Geometry check sheet. Reference: the model listing, model coordinates, mm. Face numbers are marked on the shaded views. A direction names the side the tool comes from. Give positions to 0.01 mm unless a question says otherwise; leave off trailing zeros. Order: outer loops, then holes, each group sorted by start corner. A loop starts at its lowest first (then second) coordinate and runs counter-clockwise, first axis right, second up.
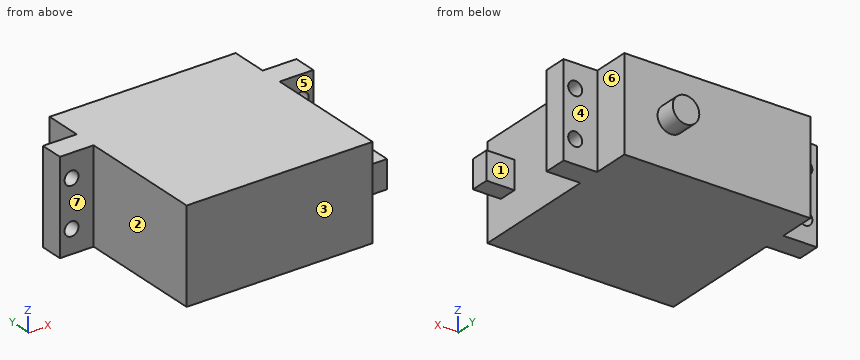
```python
from build123d import *

# Parameters (mm, degrees)
SKETCH1_W           = 40
SKETCH1_H           = 8
SKETCH1_W_2         = 7.25
SKETCH1_H_2         = 5
SKETCH1_H_3         = 27.5
BOSS_EXTRUDE1_DEPTH = 20
SKETCH2_R           = 2.85
BOSS_EXTRUDE2_DEPTH = 4.5
SKETCH3_R           = 1.5
CUT_EXTRUDE1_DEPTH  = 47.891497097
SKETCH4_W           = 6
SKETCH4_H           = 4
BOSS_EXTRUDE3_DEPTH = 6


with BuildPart() as part:
    # Sketch1 → Boss-Extrude1 (new body)
    with BuildSketch(Plane.XY):
        with Locations((0, -4)):
            Rectangle(SKETCH1_W, SKETCH1_H)
        with Locations((-23.625, -10.5)):
            Rectangle(SKETCH1_W_2, SKETCH1_H_2)
        with Locations((0, -10.5)):
            Rectangle(SKETCH1_W, SKETCH1_H_2)
        with Locations((23.625, -10.5)):
            Rectangle(SKETCH1_W_2, SKETCH1_H_2)
        with Locations((0, -26.75)):
            Rectangle(SKETCH1_W, SKETCH1_H_3)
    extrude(amount=BOSS_EXTRUDE1_DEPTH)

    # Sketch2 → Boss-Extrude2 (add)
    with BuildSketch(Plane(origin=(0, 0, 0), x_dir=(1, 0, 0), z_dir=(0, 1, 0))):
        with Locations(Location((10, -10, 0), (0, 0, 90))):
            Circle(SKETCH2_R)
    extrude(amount=BOSS_EXTRUDE2_DEPTH)

    # Sketch3 → Cut-Extrude1 (cut, through all)
    with BuildSketch(Plane(origin=(0, -8, 0), x_dir=(1, 0, 0), z_dir=(0, 1, 0))):
        with Locations(Location((-24.75, -5, 0), (0, 0, 180))):
            Circle(SKETCH3_R)
        with Locations(Location((-24.75, -15, 0), (0, 0, 180))):
            Circle(SKETCH3_R)
        with Locations(Location((24.75, -15, 0), (0, 0, 180))):
            Circle(SKETCH3_R)
        with Locations(Location((24.75, -5, 0), (0, 0, 180))):
            Circle(SKETCH3_R)
    extrude(amount=-CUT_EXTRUDE1_DEPTH, mode=Mode.SUBTRACT)

    # Sketch4 → Boss-Extrude3 (add)
    with BuildSketch(Plane(origin=(20, 0, 0), x_dir=(0, 0, -1), z_dir=(1, 0, 0))):
        with Locations((-10, -34.5)):
            Rectangle(SKETCH4_W, SKETCH4_H)
    extrude(amount=BOSS_EXTRUDE3_DEPTH)


solid = part.part
```
Q1. Cross-section at D-D, the plane z = 10. Record the boundary of the cut face in (x, y).
Q2. Release check for a two-part mould opening along Y. For the marked faces 1, 2, 3 and 4 record: pulls with the +Y half, pulls with the -Y half, needs draft (parallel to the pull), parting line crosses it, or undercut.
Q3. Cross-section at A-A, the plane z = 5. Record the boundary of the cut face in (x, y).
Q4. Cross-section at C-C, the plane x = 24.75. Record the boundary of the cut face in (y, z).
Q5. Access from +Z, -Z, +X, -X, +Y, -Y to the whole of each face (thin tool, end or side, straight path). Record for the marked faces 5, 6 and 7.
Q6. Cross-section at B-B, the plane y = -11.5. Record the boundary of the cut face in (x, z).
Q7. Gauge pin test, flat ends, axial feed: P1, Ø1.5, axis at y = -4.5, z = 4, coming from the +X side; P2, Ø3.5, axis at x = 23.5, z = 12, coming from the +Y side; P3, Ø1.2, axis at x = 22.5, y = -34.5, coming from the -Z side. Record the tip position at first contact, or that the pin passes through.
Q8. Thickness scan on L1, parallel to Z at x = 24, y = -10; L2, parallel to Y at x = -23, z = 9.5; L3, parallel to Y at x = 12, z = 3.5. Record the ranges inside material, lowest first.
Answers follow:
1. outline: (-27.25, -13) - (-20, -13) - (-20, -40.5) - (20, -40.5) - (20, -36.5) - (26, -36.5) - (26, -32.5) - (20, -32.5) - (20, -13) - (27.25, -13) - (27.25, -8) - (20, -8) - (20, 0) - (12.85, 0) - (12.85, 4.5) - (7.15, 4.5) - (7.15, 0) - (-20, 0) - (-20, -8) - (-27.25, -8) - close
2. face 1: undercut
2. face 2: needs draft
2. face 3: pulls with the -Y half
2. face 4: pulls with the +Y half
3. outline: (-27.25, -13) - (-26.25, -13) - (-26.25, -8) - (-27.25, -8) - close; (-23.25, -13) - (-20, -13) - (-20, -40.5) - (20, -40.5) - (20, -13) - (23.25, -13) - (23.25, -8) - (20, -8) - (20, 0) - (-20, 0) - (-20, -8) - (-23.25, -8) - close; (26.25, -13) - (27.25, -13) - (27.25, -8) - (26.25, -8) - close
4. outline: (-36.5, 7) - (-32.5, 7) - (-32.5, 13) - (-36.5, 13) - close; (-13, 0) - (-8, 0) - (-8, 3.5) - (-13, 3.5) - close; (-13, 6.5) - (-8, 6.5) - (-8, 13.5) - (-13, 13.5) - close; (-13, 16.5) - (-8, 16.5) - (-8, 20) - (-13, 20) - close
5. face 5: +Z, -Z, +X
5. face 6: +Z, -Z, +X, +Y
5. face 7: +Z, -Z, -X, -Y
6. outline: (-27.25, 0) - (27.25, 0) - (27.25, 20) - (-27.25, 20) - close; hole circle Ø3 at (-24.75, 5); hole circle Ø3 at (-24.75, 15); hole circle Ø3 at (24.75, 5); hole circle Ø3 at (24.75, 15)
7. P1: stops at x = 20
7. P2: stops at y = -8
7. P3: stops at z = 7
8. L1: z = 0 to 3.7, 6.3 to 13.7, 16.3 to 20
8. L2: y = -13 to -8
8. L3: y = -40.5 to 0
